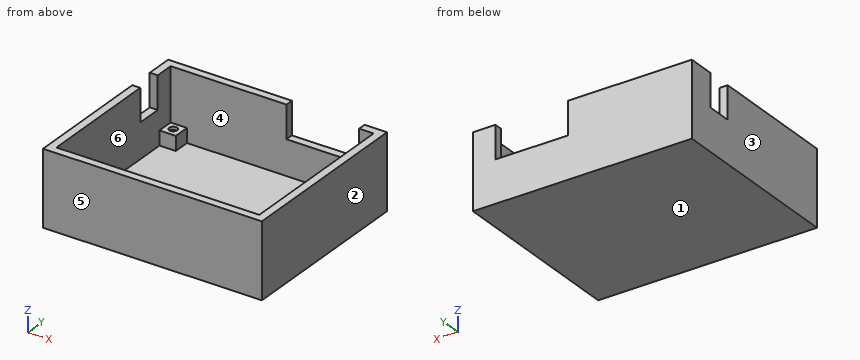
from build123d import *

# Parameters (mm, degrees)
ESBO_O1_W                = 107
ESBO_O1_H                = 89.6
RESSALTO_EXTRUS_O2_DEPTH = 36.5
CORTE_EXTRUS_O2_DEPTH    = 33
ESBO_O4_W                = 8
ESBO_O4_H                = 8
CORTE_EXTRUS_O3_DEPTH    = 26
ESBO_O5_W                = 83.2
ESBO_O5_H                = 3.9
ESBO_O5_H_2              = 4.1
CORTE_EXTRUS_O4_DEPTH    = 33
ESBO_O6_W                = 83.2
ESBO_O6_H                = 3.9
CORTE_EXTRUS_O5_DEPTH    = 33
ESBO_O7_W                = 35.5
ESBO_O7_H                = 3.9
CORTE_EXTRUS_O6_DEPTH    = 16
ESBO_O9_W                = 3.9
ESBO_O9_H                = 12.5
CORTE_EXTRUS_O7_DEPTH    = 16
ESBO_O10_R               = 1.95
CORTE_EXTRUS_O8_DEPTH    = 1.5
ESBO_O11_R               = 1.95
CORTE_EXTRUS_O9_DEPTH    = 1.5
ESBO_O12_R               = 1.95
CORTE_EXTRUS_O10_DEPTH   = 1.5
ESBO_O13_R               = 1.95
CORTE_EXTRUS_O11_DEPTH   = 1.5
ESBO_O14_R               = 1.5
CORTE_EXTRUS_O12_DEPTH   = 7
ESBO_O15_R               = 1.5
CORTE_EXTRUS_O13_DEPTH   = 7
ESBO_O16_R               = 1.5
CORTE_EXTRUS_O14_DEPTH   = 7
ESBO_O17_R               = 1.5
CORTE_EXTRUS_O15_DEPTH   = 7


with BuildPart() as part:
    # Esboço1 → Ressalto-extrusão2 (new body)
    with BuildSketch(Plane.XY):
        with Locations((53.5, -44.8)):
            Rectangle(ESBO_O1_W, ESBO_O1_H)
    extrude(amount=RESSALTO_EXTRUS_O2_DEPTH)

    # Esboço3 → Corte-extrusão2 (cut)
    with BuildSketch(Plane.XY.offset(36.5)):
        Polygon((95.1, -77.7), (95.1, -81.8), (11.9, -81.8), (11.9, -77.7), (7.8, -77.7), (3.9, -77.7), (3.9, -11.9), (11.9, -11.9), (11.9, -7.8), (95.1, -7.8), (95.1, -11.9), (99.2, -11.9), (103.1, -11.9), (103.1, -77.7), (99.2, -77.7), align=None)
    extrude(amount=-CORTE_EXTRUS_O2_DEPTH, mode=Mode.SUBTRACT)

    # Esboço4 → Corte-extrusão3 (cut)
    with BuildSketch(Plane.XY.offset(36.5)):
        Polygon((3.9, -11.9), (3.9, -3.9), (11.9, -3.9), (11.9, -7.8), (11.9, -11.9), align=None)
        Polygon((103.1, -11.9), (103.1, -3.9), (95.1, -3.9), (95.1, -7.8), (95.1, -11.9), align=None)
        with Locations((7.9, -81.7)):
            Rectangle(ESBO_O4_W, ESBO_O4_H)
        with Locations((99.1, -81.7)):
            Rectangle(ESBO_O4_W, ESBO_O4_H)
    extrude(amount=-CORTE_EXTRUS_O3_DEPTH, mode=Mode.SUBTRACT)

    # Esboço5 → Corte-extrusão4 (cut)
    with BuildSketch(Plane.XY.offset(36.5)):
        with Locations((53.5, -5.85)):
            Rectangle(ESBO_O5_W, ESBO_O5_H)
        with Locations((53.5, -79.75)):
            Rectangle(ESBO_O5_W, ESBO_O5_H_2)
    extrude(amount=-CORTE_EXTRUS_O4_DEPTH, mode=Mode.SUBTRACT)

    # Esboço6 → Corte-extrusão5 (cut)
    with BuildSketch(Plane.XY.offset(36.5)):
        with Locations((53.5, -83.75)):
            Rectangle(ESBO_O6_W, ESBO_O6_H)
    extrude(amount=-CORTE_EXTRUS_O5_DEPTH, mode=Mode.SUBTRACT)

    # Esboço7 → Corte-extrusão6 (cut)
    with BuildSketch(Plane.XY.offset(36.5)):
        with Locations((78.25, -1.95)):
            Rectangle(ESBO_O7_W, ESBO_O7_H)
    extrude(amount=-CORTE_EXTRUS_O6_DEPTH, mode=Mode.SUBTRACT)

    # Esboço9 → Corte-extrusão7 (cut)
    with BuildSketch(Plane.XY.offset(36.5)):
        with Locations((1.95, -19.41)):
            Rectangle(ESBO_O9_W, ESBO_O9_H)
    extrude(amount=-CORTE_EXTRUS_O7_DEPTH, mode=Mode.SUBTRACT)

    # Esboço10 → Corte-extrusão8 (cut)
    with BuildSketch(Plane.XY.offset(10.5)):
        with Locations((7.8, -7.8)):
            Circle(ESBO_O10_R)
    extrude(amount=-CORTE_EXTRUS_O8_DEPTH, mode=Mode.SUBTRACT)

    # Esboço11 → Corte-extrusão9 (cut)
    with BuildSketch(Plane.XY.offset(10.5)):
        with Locations((99.2, -7.8)):
            Circle(ESBO_O11_R)
    extrude(amount=-CORTE_EXTRUS_O9_DEPTH, mode=Mode.SUBTRACT)

    # Esboço12 → Corte-extrusão10 (cut)
    with BuildSketch(Plane.XY.offset(10.5)):
        with Locations((99.2, -81.8)):
            Circle(ESBO_O12_R)
    extrude(amount=-CORTE_EXTRUS_O10_DEPTH, mode=Mode.SUBTRACT)

    # Esboço13 → Corte-extrusão11 (cut)
    with BuildSketch(Plane.XY.offset(10.5)):
        with Locations((7.8, -81.8)):
            Circle(ESBO_O13_R)
    extrude(amount=-CORTE_EXTRUS_O11_DEPTH, mode=Mode.SUBTRACT)

    # Esboço14 → Corte-extrusão12 (cut)
    with BuildSketch(Plane.XY.offset(9)):
        with Locations((7.8, -7.8)):
            Circle(ESBO_O14_R)
    extrude(amount=-CORTE_EXTRUS_O12_DEPTH, mode=Mode.SUBTRACT)

    # Esboço15 → Corte-extrusão13 (cut)
    with BuildSketch(Plane.XY.offset(9)):
        with Locations((99.2, -7.8)):
            Circle(ESBO_O15_R)
    extrude(amount=-CORTE_EXTRUS_O13_DEPTH, mode=Mode.SUBTRACT)

    # Esboço16 → Corte-extrusão14 (cut)
    with BuildSketch(Plane.XY.offset(9)):
        with Locations((99.2, -81.8)):
            Circle(ESBO_O16_R)
    extrude(amount=-CORTE_EXTRUS_O14_DEPTH, mode=Mode.SUBTRACT)

    # Esboço17 → Corte-extrusão15 (cut)
    with BuildSketch(Plane.XY.offset(9)):
        with Locations((7.8, -81.8)):
            Circle(ESBO_O17_R)
    extrude(amount=-CORTE_EXTRUS_O15_DEPTH, mode=Mode.SUBTRACT)


solid = part.part
The model under review builds one solid part; all positions refer to its coordinate system, in mm. Face numbers are marked on the shaded views. A direction names the side the tool comes from. Coordinates: 2 decimals unless noted, no trailing zeros. Write each loop counter-clockwise with the first axis right and the second up, starting at its lowest first coordinate (ties: lowest second). Pieces come first, ordered by that corner, then holes. Notation, with made-up numbers: M -19.5,52.5 L 23.5,52.5 A20 ccw 23.5,75.5 Z; hole C 17,61.5 d3. An arc over 180 degrees is marked long. Put each result on its own line as item: value.
1) Add section A-A on z = 12.5. Give the boundary of the cut face in (x, y).
Computed:
outline: M 0,-89.6 L 107,-89.6 L 107,0 L 0,0 Z; hole M 3.9,-85.7 L 103.1,-85.7 L 103.1,-3.9 L 3.9,-3.9 Z
2) Draft analysis for pull direction X (two halves, no side actions). For the marked faces 1, 2, 3 and 4, state which applies: released by +X, released by -X, zero draft, split by the parting line, or undercut.
Computed:
face 1: zero draft
face 2: released by +X
face 3: released by -X
face 4: undercut
3) Add section D-D on x = 70. Give the boundary of the cut face in (y, z), then the cut area to 3 significant figures.
Computed:
outline: M -89.6,0 L 0,0 L 0,20.5 L -3.9,20.5 L -3.9,3.5 L -85.7,3.5 L -85.7,36.5 L -89.6,36.5 Z
area: 509 mm2
4) For the marked faces 5 and 6, list the 3-axis set-ups (+Z, -Z, +X, -X, +Y, -Y) from which the entire face can be reached by the end or side of a thin tool; tool diameter is ignored.
Computed:
face 5: +Z, -Z, +X, -X, -Y
face 6: +Z
5) Add section C-C on y = -38. Give the boundary of the cut face in (x, z).
Computed:
outline: M 0,0 L 107,0 L 107,36.5 L 103.1,36.5 L 103.1,3.5 L 3.9,3.5 L 3.9,36.5 L 0,36.5 Z
6) Wall thickness on probe 1 along Y at (x, z) = (99.2, 4); probe 2 along Y at (x, z) = (7.8, 9.95); probe 3 along X at (y, z) = (-81.8, 4): over which ranges is each line inside the solid? List them lowest first. Write a range as [from, to].
Computed:
probe 1: y = [-89.6, -83.3], [-80.3, -77.7], [-11.9, -9.3], [-6.3, 0]
probe 2: y = [-89.6, -83.75], [-79.85, -77.7], [-11.9, -9.75], [-5.85, 0]
probe 3: x = [0, 6.3], [9.3, 11.9], [95.1, 97.7], [100.7, 107]
7) Clearance check with flat-ended pins moving along their axes: pin 1 Ø3 at (x, y) = (8, -81.5) entering from +Z; pin 2 Ø3 at (x, y) = (69.5, -2) entering from +Z; pin 3 Ø4 at (x, y) = (8, -83.5) entering from +Z. State where each tip first meets the part, or that it passes through.
Computed:
pin 1: stops at z = 9
pin 2: stops at z = 20.5
pin 3: stops at z = 10.5
8) Add section B-B on z = 6.5. Give the boundary of the cut face in (x, y), then the cut area to 3 significant figures.
Computed:
outline: M 0,-89.6 L 107,-89.6 L 107,0 L 0,0 Z; hole M 3.9,-77.7 L 11.9,-77.7 L 11.9,-85.7 L 95.1,-85.7 L 95.1,-77.7 L 103.1,-77.7 L 103.1,-11.9 L 95.1,-11.9 L 95.1,-3.9 L 11.9,-3.9 L 11.9,-11.9 L 3.9,-11.9 Z; hole C 7.8,-81.8 d3; hole C 7.8,-7.8 d3; hole C 99.2,-81.8 d3; hole C 99.2,-7.8 d3
area: 1,700 mm2
